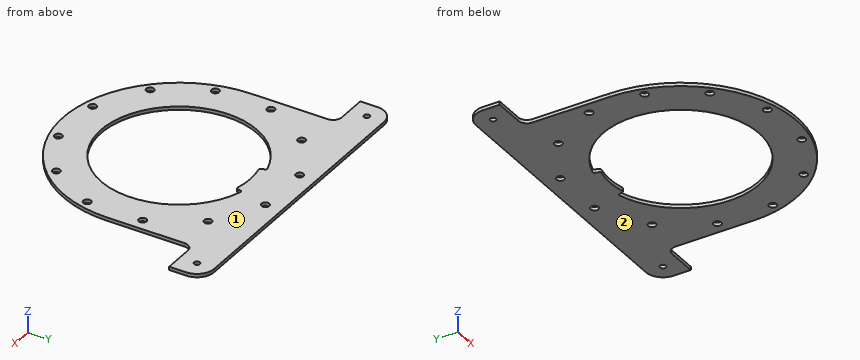
Autodesk Inventor part; units mm, degrees
ref_plane "YZ Plane" through (0, 0, 0) normal (1, 0, 0) x (0, 1, 0)
ref_plane "XZ Plane" through (0, 0, 0) normal (0, 1, 0) x (-1, 0, 0)
ref_plane "XY Plane" through (0, 0, 0) normal (0, 0, 1) x (1, 0, 0)
sketch "スケッチ1" plane through (0, 0, 0) normal (0, 0, 1) x (1, 0, 0)
  line L0 (-90, -67.5) -> (90, -67.5)
  line L1 (90, -67.5) -> (90, 70)
  line L2 (90, 70) -> (-90, 70)
  line L3 (-90, 70) -> (-90, -67.5)
  point P0 (0, 0)
  point P1 (-29.0861, -67.5)
  dimension "d37" = 90
  dimension "d38" = 70
  dimension "d40" = 90
  dimension "d41" = 67.5
extrude "プレート1" add sketch "スケッチ1" along normal blind 2
sketch "スケッチ2" plane through (0, 0, 2) normal (0, 0, 1) x (1, 0, 0)
  circle A0 centre (0, 0) radius 45.5
  dimension "d5" = 91
extrude "押し出し1" cut sketch "スケッチ2" against normal blind 10
sketch "スケッチ3" plane through (0, 0, 2) normal (0, 0, 1) x (1, 0, 0)
  circle A0 centre (0, 0) radius 62.5
  point P0 (-16.1762, 60.3704)
  point P1 (-44.1942, 44.1942)
  point P2 (-60.3704, 16.1762)
  point P3 (-60.3704, -16.1762)
  point P4 (-44.1942, -44.1942)
  point P5 (-16.1762, -60.3704)
  point P6 (16.1762, -60.3704)
  point P7 (44.1942, -44.1942)
  point P8 (60.3704, -16.1762)
  point P9 (60.3704, 16.1762)
  point P10 (44.1942, 44.1942)
  point P11 (16.1762, 60.3704)
  dimension "d8" = 125
  dimension "d11" = 360
  dimension "d20" = 0
hole "穴1" at (-16.1762, 60.3704, 2) at (-44.1942, 44.1942, 2) at (-60.3704, 16.1762, 2) at (-60.3704, -16.1762, 2) at (-44.1942, -44.1942, 2) at (-16.1762, -60.3704, 2) at (16.1762, -60.3704, 2) at (44.1942, -44.1942, 2) at (60.3704, -16.1762, 2) at (60.3704, 16.1762, 2) at (44.1942, 44.1942, 2) at (16.1762, 60.3704, 2) direction (0, 0, -1) diameter 4.5 end through all
fillet "コーナーR2" radius 10 2 edges at (-90, 70, 1) (90, 70, 1)
sketch "スケッチ5" plane through (0, 0, 2) normal (0, 0, 1) x (1, 0, 0)
  arc A0 (-80, 70) -> (-90, 60) centre (-80, 60) ccw
  arc A1 (90, 60) -> (80, 70) centre (80, 60) ccw
  point P0 (0, 0)
hole "穴2" at (-80, 60, 2) at (80, 60, 2) direction (0, 0, -1) diameter 3.4 end through all
sketch "スケッチ7" plane through (0, 0, 2) normal (0, 0, 1) x (1, 0, 0)
  circle A0 centre (0, 0) radius 45.5
  circle A1 centre (0, 0) radius 67.5
  line L0 (90, -67.5) -> (-90, -67.5)
  line L1 (-90, -67.5) -> (-90, 60)
  line L2 (-90, -67.5) -> (-67.5, -67.5)
  line L3 (-67.5, -67.5) -> (-67.5, 50)
  line L4 (-67.5, 50) -> (-90, 50)
  line L5 (-90, 50) -> (-90, -67.5)
  line L6 (90, -67.5) -> (67.5, -67.5)
  line L7 (67.5, -67.5) -> (67.5, 50)
  line L8 (67.5, 50) -> (90, 50)
  line L9 (90, 50) -> (90, -67.5)
  line L10 (-80, 70) -> (80, 70)
  point P0 (67.5, 0)
  point P1 (0, -67.5)
  point P2 (-67.5, 0)
  dimension "d56" = 20
  dimension "d57" = 20
extrude "押し出し4" cut sketch "スケッチ7" against normal blind 10 contours L7 L0 A1 | L7 L8 L9 L0 | A1 L0 L3 | L3 L0 L1 L4
fillet "コーナーR4" radius 5 2 edges at (-67.5, 50, 1) (67.5, 50, 1)
sketch "スケッチ9" plane through (0, 0, 2) normal (0, 0, 1) x (1, 0, 0)
  circle A0 centre (0, 0) radius 45.5
  circle A1 centre (0, 0) radius 41.5
  line L0 (0, 0) -> (-11.7763, 43.9496)
  line L1 (11.7763, 43.9496) -> (0, 0)
  line L2 (0, 97.5) -> (0, -95)
  point P0 (-10.741, 40.0859)
  point P1 (10.741, 40.0859)
  dimension "d76" = 4
  dimension "d77" = 15
  dimension "d78" = 15
extrude "押し出し5" add sketch "スケッチ9" against normal up to surface (2 mm away) contours L1 A1 L2 A0 | L2 A1 L0 A0 picked at (5.1612, 43.8259) picked at (-6.3577, 43.6684)
fillet "コーナーR5" radius 1 4 edges at (10.741, 40.0859, 1) (-10.741, 40.0859, 1) (-11.7763, 43.9496, 1) (11.7763, 43.9496, 1)
equation "\"d18\" = Thickness"
equation "\"d47\" = Thickness"
equation "\"d2\" = Thickness"
equation "\"BendRadius\" = Thickness"
equation "\"BendReliefWidth\" = Thickness"
equation "\"BendReliefDepth\" = 0.5 * Thickness"
equation "\"CornerReliefSize\" = 4 * Thickness"
equation "\"MinimumRemnant\" = 2 * Thickness"
equation "\"TransitionRadius\" = BendRadius"
equation "\"JacobiRadiusSize\" = BendRadius"
equation "\"GapSize\" = Thickness"
properties part number "base4" material "CFRP"
The listing builds one solid part. Answer for the finished solid, in the listing's coordinates (mm). Face numbers are marked on the shaded views. Round coordinates to 2 decimals unless told otherwise and drop trailing zeros. Write each loop counter-clockwise with the first axis right and the second up, starting at its lowest first coordinate (ties: lowest second). Pieces come first, ordered by that corner, then holes. Notation, with made-up numbers: (-21, 52.25) - (-4, 52.25) arc R18 cw to (-4, 87.25) - close; hole circle Ø2 at (66, 33.5). An arc over 180 degrees is marked (long way). Use a Markdown table: item, result. Add a question column.
1. The part is cut by section D-D (x = 75). Write down the section's boundary in (y, z).
2. Flat-ended cylindrical pins translate along their axes: P1, Ø2.5, axis at x = -80, y = 60, coming from the +Z side; P2, Ø1, axis at x = -80.5, z = 1, coming from the -Y side. Find the tip coordinate at first contact, or state that the pin passes through.
3. The part is cut by section B-B (y = 7). Write down the section's boundary in (x, z).
4. The part is cut by section C-C (z = 1.2). Give the number of separate pieces and of enclosed holes in the cut face, and give its area (3 significant figures).
5. For a pull along Z with two mould halves and no side action, classify the marked faces 1 and 2 as +Z half, -Z half, draft (parallel to the pull), parting line (faces both ways), or undercut.
6. The part is cut by section A-A (x = 0). Write down the section's boundary in (y, z).
7. Consider line 1 (X direction, y = 62, z = 1.65); line 2 (X direction, y = 0, z = 0.7); line 3 (X direction, y = 60, z = 1.55). Determine where each line is inside the solid, lowest interval first.
Reported:
| question | item | result |
|---|---|---|
| 1 | outline | (50, 0) - (70, 0) - (70, 2) - (50, 2) - close |
| 2 | P1 | through |
| 2 | P2 | y = 50 |
| 3 | outline | (-67.5, 0) - (-44.96, 0) - (-44.96, 2) - (-67.5, 2) - close; (44.96, 0) - (67.5, 0) - (67.5, 2) - (44.96, 2) - close |
| 4 | separate pieces | 1 |
| 4 | enclosed holes | 15 |
| 4 | area | 10,900 mm^2 |
| 5 | face 1 | +Z half |
| 5 | face 2 | -Z half |
| 6 | outline | (-67.5, 0) - (-45.5, 0) - (-45.5, 2) - (-67.5, 2) - close; (41.5, 0) - (70, 0) - (70, 2) - (41.5, 2) - close |
| 7 | line 1 | -89.8 to -17.73, -14.62 to 14.62, 17.73 to 89.8 |
| 7 | line 2 | -67.5 to -45.5, 45.5 to 67.5 |
| 7 | line 3 | -90 to -81.7, -78.3 to -18.4, -13.96 to 13.96, 18.4 to 78.3, 81.7 to 90 |
